Autodesk Inventor part; units mm, degrees
ref_plane "YZ Plane" through (0, 0, 0) normal (1, 0, 0) x (0, 1, 0)
ref_plane "XZ Plane" through (0, 0, 0) normal (0, 1, 0) x (-1, 0, 0)
ref_plane "XY Plane" through (0, 0, 0) normal (0, 0, 1) x (1, 0, 0)
sketch "Sketch1" plane through (0, 0, 0) normal (0, 1, 0) x (-1, 0, 0)
  line L0 (-27.5, 22.5) -> (27.5, 22.5)
  line L1 (27.5, 22.5) -> (27.5, -22.5)
  line L2 (27.5, -22.5) -> (-27.5, -22.5)
  line L3 (-27.5, -22.5) -> (-27.5, 22.5)
  line L4 (-27.5, 22.5) -> (27.5, -22.5) construction
  line L5 (27.5, 22.5) -> (-27.5, -22.5) construction
  point P0 (0, 0)
  dimension "d0" = 45
  dimension "d1" = 55
extrude "Extrusion1" add sketch "Sketch1" along normal mid plane 8.763
sketch "Sketch2" plane through (0, 4.3815, 0) normal (0, 1, 0) x (1, 0, 0)
  line L0 (-27.5, -22.5) -> (27.5, -22.5)
  line L1 (27.5, -22.5) -> (27.5, 22.5)
  point P0 (4.8, -9.8)
  dimension "d11" = 12.7
  dimension "d12" = 22.7
hole "Hole1" at (4.8, 4.3815, 9.8) direction (0, -1, 0) diameter 4.496 end through all
sketch "Sketch3" plane through (0, 4.3815, 0) normal (0, 1, 0) x (1, 0, 0)
  line L0 (27.5, 22.5) -> (-27.5, 22.5)
  line L1 (-27.5, 22.5) -> (-12.5, 22.5)
  line L2 (-12.5, 22.5) -> (-12.5, -22.5)
  line L3 (-12.5, -22.5) -> (-27.5, -22.5)
  line L4 (-27.5, -22.5) -> (-27.5, 22.5)
  line L5 (-27.5, -22.5) -> (27.5, -22.5)
  point P0 (0, 0)
  dimension "d13" = 15
extrude "Extrusion2" add sketch "Sketch3" along normal blind 31.136
sketch "Sketch9" plane through (0, -4.3815, 0) normal (0, -1, 0) x (1, 0, 0)
  circle A0 centre (4.8, 9.8) radius 2.248
  circle A1 centre (4.8, 9.8) radius 4
  point P0 (0, 0)
  dimension "d40" = 8
extrude "Extrusion8" cut sketch "Sketch9" against normal blind 4.318
sketch "Sketch10" plane through (0, -4.3815, 0) normal (0, -1, 0) x (1, 0, 0)
  line L0 (27.5, -22.5) -> (27.5, 22.5)
  line L1 (-27.5, -22.5) -> (27.5, -22.5)
  line L2 (27.5, 22.5) -> (-27.5, 22.5)
  point P0 (0, 0)
  point P1 (22.42, -7.726)
  point P2 (22.42, 17.42)
  point P3 (2.1, -7.726)
  dimension "d43" = 5.08
  dimension "d45" = 20.32
  dimension "d46" = 25.146
  dimension "d65" = 5.08
hole "Hole2" at (22.42, -4.3815, -7.726) at (22.42, -4.3815, 17.42) at (2.1, -4.3815, -7.726) direction (0, 1, 0) diameter 3.797 end through all
fillet "Fillet1" radius 2 2 edges at (27.5, 0, 22.5) (27.5, 0, -22.5)
sketch "Sketch13" plane through (0, 35.5175, 0) normal (0, 1, 0) x (1, 0, 0)
  line L0 (-12.5, 22.5) -> (-27.5, 22.5)
  point P0 (0, 0)
  point P1 (-20, 14.5)
  point P2 (-20, 22.5)
  dimension "d74" = 8
hole "Hole4" at (-20, 35.5175, -14.5) direction (0, -1, 0) diameter 2.642 end through all
sketch "Sketch14" plane through (0, 4.3815, 0) normal (0, 1, 0) x (1, 0, 0)
  line L0 (-12.5, -22.5) -> (-12.5, 22.5)
  line L1 (-12.5, -22.5) -> (-7.9, -22.5)
  line L2 (-7.9, -22.5) -> (-7.9, 2.9)
  line L3 (-7.9, 2.9) -> (-12.5, 2.9)
  line L4 (-12.5, 2.9) -> (-12.5, -22.5)
  point P0 (0, 0)
  dimension "d89" = 25.4
  dimension "d90" = 4.6
extrude "Extrusion11" add sketch "Sketch14" along normal blind 5
properties part number "BaseMount"
Geometry check sheet. Reference: the model listing, model coordinates, mm. A direction names the side the tool comes from. Give positions to 0.01 mm unless a question says otherwise; leave off trailing zeros. Order: outer loops, then holes, each group sorted by start corner. A loop starts at its lowest first (then second) coordinate and runs counter-clockwise, first axis right, second up.
1. Thickness scan on L1, parallel to Z at x = 22.42, y = 1; L2, parallel to Z at x = 2, y = 2; L3, parallel to X at y = 0.25, z = 17.42. Record the ranges inside material, lowest first.
2. Section check D-D, the plane x = 22.42. Enter the section's corners in (y, z).
3. Access from +Z, -Z, +X, -X, +Y, -Y to the whole of each face (thin tool, end or side, straight path). Record for faces 5 (the face through (-10, 7, -2.9)), 6 (the face through (-7.9, 7, 10)), 7 (the face through (6.95, -2.253, 13.173)), 8 (the face through (-12, 2, -22.5)).
4. Section check A-A, the plane z = 9.8. Enter the section's corners in (x, y).
5. Section check C-C, the plane y = -1. Enter the section's corners in (x, z), and give its area (3 significant figures).
6. Gauge pin test, flat ends, axial feed: pin 1 Ø2.5 at (x, z) = (6, 11) entering from -Y; pin 2 Ø1.5 at (y, z) = (13, 5.5) entering from +X; pin 3 Ø6.5 at (x, z) = (4.8, 9.8) entering from +Y; pin 4 Ø3.5 at (x, z) = (22.42, -7.726) entering from +Y. Record the tip position at first contact, or that the pin passes through.
7. Release check for a two-part mould opening along X. For faces 1 (the face through (20.54, 0.06, 17.67)), 2 (the face through (8, 4.382, 0)), 3 (the face through (6.794, 2.128, 10.837)), 4 (the face through (26.93, 0.06, -21.9)) record: pulls with the +X half, pulls with the -X half, needs draft (parallel to the pull), parting line crosses it, or undercut.
8. Section check B-B, the plane x = 4.8. Enter the section's corners in (y, z).
Values follow:
1. L1: z = -22.5 to -9.62, -5.83 to 15.52, 19.32 to 22.5
1. L2: z = -22.5 to -9.62, -5.83 to 22.5
1. L3: x = -27.5 to 20.52, 24.32 to 27.5
2. outline: (-4.38, -22.5) - (4.38, -22.5) - (4.38, -9.62) - (-4.38, -9.62) - close; (-4.38, -5.83) - (4.38, -5.83) - (4.38, 15.52) - (-4.38, 15.52) - close; (-4.38, 19.32) - (4.38, 19.32) - (4.38, 22.5) - (-4.38, 22.5) - close
3. face 5: -Z, +X, +Y
3. face 6: +Z, -Z, +X, +Y
3. face 7: -Y
3. face 8: -Z, +X, -X, +Y, -Y
4. outline: (-27.5, -4.38) - (0.8, -4.38) - (0.8, -0.06) - (2.55, -0.06) - (2.55, 4.38) - (-7.9, 4.38) - (-7.9, 9.38) - (-12.5, 9.38) - (-12.5, 35.52) - (-27.5, 35.52) - close; (7.05, -0.06) - (8.8, -0.06) - (8.8, -4.38) - (27.5, -4.38) - (27.5, 4.38) - (7.05, 4.38) - close
5. outline: (-27.5, -22.5) - (25.5, -22.5) arc R2 ccw to (27.5, -20.5) - (27.5, 20.5) arc R2 ccw to (25.5, 22.5) - (-27.5, 22.5) - close; hole circle Ø2.64 at (-20, -14.5); hole circle Ø3.8 at (2.1, -7.73); hole circle Ø8 at (4.8, 9.8); hole circle Ø3.8 at (22.42, -7.73); hole circle Ø3.8 at (22.42, 17.42)
5. area: 2,380 mm2
6. pin 1: stops at y = -0.06
6. pin 2: stops at x = -12.5
6. pin 3: stops at y = 4.38
6. pin 4: passes through
7. face 1: undercut
7. face 2: needs draft
7. face 3: undercut
7. face 4: pulls with the +X half
8. outline: (-4.38, -22.5) - (4.38, -22.5) - (4.38, 7.55) - (-0.06, 7.55) - (-0.06, 5.8) - (-4.38, 5.8) - close; (-4.38, 13.8) - (-0.06, 13.8) - (-0.06, 12.05) - (4.38, 12.05) - (4.38, 22.5) - (-4.38, 22.5) - close
